CAD build for the part. Positions are in the model's coordinates, mm. Face numbers are marked on the shaded views. A direction names the side the tool comes from. Round coordinates to 2 decimals unless told otherwise and drop trailing zeros. Loops run counter-clockwise (first coordinate to the right, second up) from the corner with the lowest first, then second, coordinate; pieces in that order, holes last. Notation, with made-up numbers: M 23.25,83.5 L 62.25,83.5 A17 cw 62.25,109.5 Z; hole C -27.75,68.25 d2. An arc over 180 degrees is marked long. Use one line per item in the form item = value.
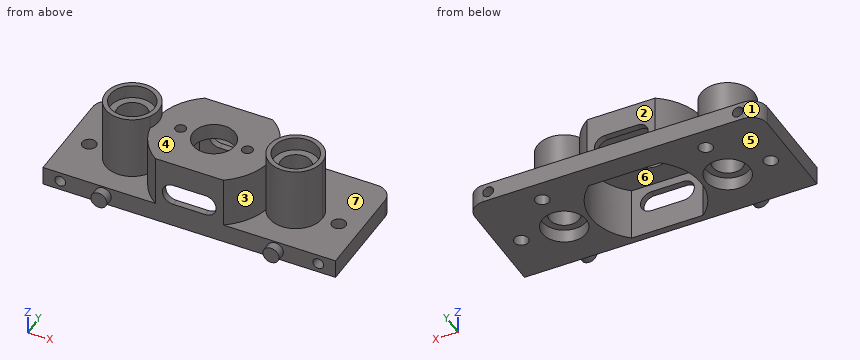
from build123d import *

# Parameters (mm, degrees)
SKETCH_2_R               = 3.9
SKETCH_2_R_2             = 4.1
SKETCH_2_R_3             = 1
SKETCH_2_R_4             = 1.3
EXTRUDE_1_DEPTH          = 3.5
SKETCH_2_4_R             = 4.1
SKETCH_2_4_R_2           = 2.8
EXTRUDE_2_DEPTH          = 1
CUT_EXTRUDE_1_DEPTH      = 41.636067723
CUT_EXTRUDE_1_DEPTH_BACK = 41.636067723
SKETCH_3_W               = 54.4
SKETCH_3_H               = 21
FILLET_1_R               = 3
CUT_EXTRUDE_2_DEPTH      = 35.541134897
CUT_EXTRUDE_2_DEPTH_BACK = 7
SKETCH_4_R               = 1
SKETCH_4_4_R             = 1.5
EXTRUDE_3_DEPTH          = 1.6
SKETCH_5_R               = 1
SKETCH_5_R_2             = 3.9
EXTRUDE_4_DEPTH          = 13
SKETCH_6_R               = 1
SKETCH_6_R_2             = 3.9
CUT_EXTRUDE_3_DEPTH      = 10
CUT_EXTRUDE_4_DEPTH      = 36.958309193
CUT_EXTRUDE_4_DEPTH_BACK = 36.958309193
SKETCH_2_5_R             = 4.1
SKETCH_2_5_R_2           = 2.8
EXTRUDE_5_DEPTH          = 13
SKETCH_8_R               = 4.1
EXTRUDE_6_DEPTH          = 12
EXTRUDE_START            = 9.5
EXTRUDE_7_DEPTH          = 2.5
SKETCH_2_6_R             = 4.1
SKETCH_2_6_R_2           = 2.8
CUT_EXTRUDE_10_DEPTH     = 2.5
SKETCH_9_R               = 1
CUT_EXTRUDE_11_DEPTH     = 6


# Read off the part's stored shape, not the designer's step: 凸台-拉伸7
with BuildPart() as part:
    # 草图2 → 凸台-拉伸1 (new body)
    with BuildSketch(Plane.XY):
        with BuildLine():
            Line((15.2, -20), (-15.2, -20))
            ThreePointArc((-15.2, -20), (-35.2, 0), (-15.2, 20))
            Line((-15.2, 20), (15.2, 20))
            ThreePointArc((15.2, 20), (35.2, 0), (15.2, -20))
        make_face()
        Circle(SKETCH_2_R, mode=Mode.SUBTRACT)
        with Locations((-15.2, 0)):
            Circle(SKETCH_2_R_2, mode=Mode.SUBTRACT)
        with Locations((15.2, 0)):
            Circle(SKETCH_2_R_2, mode=Mode.SUBTRACT)
        with Locations((-6.2, 0)):
            Circle(SKETCH_2_R_3, mode=Mode.SUBTRACT)
        with Locations((6.2, 0)):
            Circle(SKETCH_2_R_3, mode=Mode.SUBTRACT)
        with Locations((-15.2, 8)):
            Circle(SKETCH_2_R_4, mode=Mode.SUBTRACT)
        with Locations((-23.2, 0)):
            Circle(SKETCH_2_R_4, mode=Mode.SUBTRACT)
        with Locations((23.2, 0)):
            Circle(SKETCH_2_R_4, mode=Mode.SUBTRACT)
        with Locations((15.2, 8)):
            Circle(SKETCH_2_R_4, mode=Mode.SUBTRACT)
    extrude(amount=EXTRUDE_1_DEPTH)

    # 草图2<4> → 凸台-拉伸2 (add)
    # profile 1 of 2: a face of its own
    with BuildSketch(Plane.XY):
        with Locations((-15.2, 0)):
            Circle(SKETCH_2_4_R)
        with Locations((-15.2, 0)):
            Circle(SKETCH_2_4_R_2, mode=Mode.SUBTRACT)
    # profile 2 of 2: a face of its own
    with BuildSketch(Plane.XY):
        with Locations((15.2, 0)):
            Circle(SKETCH_2_4_R)
        with Locations((15.2, 0)):
            Circle(SKETCH_2_4_R_2, mode=Mode.SUBTRACT)
    extrude(amount=EXTRUDE_2_DEPTH)

    # 草图3 → 切除-拉伸1 (cut, two sides: drawn at the far end of the back side and taken through both)
    with BuildSketch(Plane.XY.offset(3.5).offset(-CUT_EXTRUDE_1_DEPTH_BACK)):
        with BuildLine():
            Line((15.2, -20), (-15.2, -20))
            ThreePointArc((-15.2, -20), (-35.2, 0), (-15.2, 20))
            Line((-15.2, 20), (15.2, 20))
            ThreePointArc((15.2, 20), (35.2, 0), (15.2, -20))
        make_face()
        with Locations((0, 1.5)):
            Rectangle(SKETCH_3_W, SKETCH_3_H, mode=Mode.SUBTRACT)
    extrude(amount=CUT_EXTRUDE_1_DEPTH + CUT_EXTRUDE_1_DEPTH_BACK, mode=Mode.SUBTRACT)

    # 圆角1
    fillet_1_edges = [part.edges().sort_by_distance(p)[0] for p in [
        (27.2, 12, 1.75),
        (-27.2, 12, 1.75),
    ]]
    fillet(fillet_1_edges, radius=FILLET_1_R)

    # 草图4 → 切除-拉伸2 (cut, two sides: drawn at the far end of the back side and taken through both)
    with BuildSketch(Plane.XZ.offset(9).offset(-CUT_EXTRUDE_2_DEPTH_BACK)):
        with Locations(Location((-24, 1.75, 0), (0, 0, 90))):
            Circle(SKETCH_4_R)
        with Locations(Location((24, 1.75, 0), (0, 0, 90))):
            Circle(SKETCH_4_R)
    extrude(amount=CUT_EXTRUDE_2_DEPTH + CUT_EXTRUDE_2_DEPTH_BACK, mode=Mode.SUBTRACT)

    # 草图4<4> → 凸台-拉伸3 (add)
    with BuildSketch(Plane.XZ.offset(9)):
        with Locations(Location((-16, 1.75, 0), (0, 0, 270))):
            Circle(SKETCH_4_4_R)
        with Locations(Location((16, 1.75, 0), (0, 0, 270))):
            Circle(SKETCH_4_4_R)
    extrude(amount=EXTRUDE_3_DEPTH)

    # 草图5 → 凸台-拉伸4 (add)
    with BuildSketch(Plane(origin=(0, 0, 0), x_dir=(-1, 0, 0), z_dir=(0, 0, -1))):
        with BuildLine():
            Line((6.32455532, 9), (-6.32455532, 9))
            ThreePointArc((-6.32455532, 9), (-11, 0), (-6.32455532, -9))
            Line((-6.32455532, -9), (6.32455532, -9))
            ThreePointArc((6.32455532, -9), (9.761406367, -5.070990607), (11, 0))
            ThreePointArc((11, 0), (9.761406367, 5.070990607), (6.32455532, 9))
        make_face()
        with Locations((-6.2, 0)):
            Circle(SKETCH_5_R, mode=Mode.SUBTRACT)
        Circle(SKETCH_5_R_2, mode=Mode.SUBTRACT)
        with Locations((6.2, 0)):
            Circle(SKETCH_5_R, mode=Mode.SUBTRACT)
    extrude(amount=-EXTRUDE_4_DEPTH)

    # 草图6 → 切除-拉伸3 (cut)
    with BuildSketch(Plane(origin=(0, 0, 0), x_dir=(-1, 0, 0), z_dir=(0, 0, -1))):
        with BuildLine():
            Line((6.65, 7.8), (-6.65, 7.8))
            ThreePointArc((-6.65, 7.8), (-10.25, 0), (-6.65, -7.8))
            Line((-6.65, -7.8), (6.65, -7.8))
            ThreePointArc((6.65, -7.8), (9.306583691, -4.295346319), (10.25, 0))
            ThreePointArc((10.25, 0), (9.306583691, 4.295346319), (6.65, 7.8))
        make_face()
        with Locations((-6.2, 0)):
            Circle(SKETCH_6_R, mode=Mode.SUBTRACT)
        Circle(SKETCH_6_R_2, mode=Mode.SUBTRACT)
        with Locations((6.2, 0)):
            Circle(SKETCH_6_R, mode=Mode.SUBTRACT)
    extrude(amount=-CUT_EXTRUDE_3_DEPTH, mode=Mode.SUBTRACT)

    # 草图7 → 切除-拉伸4 (cut, two sides: drawn at the far end of the back side and taken through both)
    with BuildSketch(Plane(origin=(0, 9, 0), x_dir=(1, 0, 0), z_dir=(0, 1, 0)).offset(-CUT_EXTRUDE_4_DEPTH_BACK)):
        with BuildLine():
            Line((-3, -4.5), (3, -4.5))
            ThreePointArc((3, -4.5), (5, -6.5), (3, -8.5))
            Line((3, -8.5), (-3, -8.5))
            ThreePointArc((-3, -8.5), (-5, -6.5), (-3, -4.5))
        make_face()
    extrude(amount=CUT_EXTRUDE_4_DEPTH + CUT_EXTRUDE_4_DEPTH_BACK, mode=Mode.SUBTRACT)

    # 草图2<5> → 凸台-拉伸5 (add)
    # profile 1 of 2: a face of its own
    with BuildSketch(Plane.XY):
        with Locations(Location((-15.2, 0, 0), (0, 0, 180))):
            Circle(SKETCH_2_5_R)
        with Locations((-15.2, 0)):
            Circle(SKETCH_2_5_R_2, mode=Mode.SUBTRACT)
    # profile 2 of 2: a face of its own
    with BuildSketch(Plane.XY):
        with Locations(Location((15.2, 0, 0), (0, 0, 180))):
            Circle(SKETCH_2_5_R)
        with Locations((15.2, 0)):
            Circle(SKETCH_2_5_R_2, mode=Mode.SUBTRACT)
    extrude(amount=EXTRUDE_5_DEPTH)

    # 草图8 → 凸台-拉伸6 (add)
    # profile 1 of 2: a face of its own
    with BuildSketch(Plane.XY.offset(3.5)):
        with BuildLine():
            ThreePointArc((-10.774259868, -2.217053064), (-11, 0), (-10.774259868, 2.217053064))
            ThreePointArc((-10.774259868, 2.217053064), (-20.15, 0), (-10.774259868, -2.217053064))
        make_face()
        with Locations((-15.2, 0)):
            Circle(SKETCH_8_R, mode=Mode.SUBTRACT)
    # profile 2 of 2: a face of its own
    with BuildSketch(Plane.XY.offset(3.5)):
        with BuildLine():
            ThreePointArc((10.774259868, -2.217053064), (16.339097526, -4.817152356), (20.15, 0))
            ThreePointArc((20.15, 0), (16.339097526, 4.817152356), (10.774259868, 2.217053064))
            ThreePointArc((10.774259868, 2.217053064), (11, 0), (10.774259868, -2.217053064))
        make_face()
        with Locations((15.2, 0)):
            Circle(SKETCH_8_R, mode=Mode.SUBTRACT)
    extrude(amount=EXTRUDE_6_DEPTH)

    # 凸台-拉伸7 outline → 凸台-拉伸7 (add)
    with BuildSketch(Plane.XY.offset(3.5).offset(EXTRUDE_START)):
        with BuildLine():
            ThreePointArc((-10.774259868, -2.217053064), (-10.25, 0), (-10.774259868, 2.217053064))
            ThreePointArc((-10.774259868, 2.217053064), (-11, 0), (-10.774259868, -2.217053064))
        make_face()
        with BuildLine():
            ThreePointArc((10.774259868, -2.217053064), (11, 0), (10.774259868, 2.217053064))
            ThreePointArc((10.774259868, 2.217053064), (10.25, 0), (10.774259868, -2.217053064))
        make_face()
    extrude(amount=EXTRUDE_7_DEPTH)

    # 草图2<6> → 切除-拉伸10 (cut)
    # profile 1 of 2: a face of its own
    with BuildSketch(Plane.XY):
        with Locations((-15.2, 0)):
            Circle(SKETCH_2_6_R)
        with Locations((-15.2, 0)):
            Circle(SKETCH_2_6_R_2, mode=Mode.SUBTRACT)
    # profile 2 of 2: a face of its own
    with BuildSketch(Plane.XY):
        with Locations((15.2, 0)):
            Circle(SKETCH_2_6_R)
        with Locations((15.2, 0)):
            Circle(SKETCH_2_6_R_2, mode=Mode.SUBTRACT)
    extrude(amount=CUT_EXTRUDE_10_DEPTH, mode=Mode.SUBTRACT)

    # 草图9 → 切除-拉伸11 (cut)
    with BuildSketch(Plane(origin=(0, 12, 0), x_dir=(1, 0, 0), z_dir=(0, 1, 0))):
        with Locations(Location((-23.2, -1.75, 0), (0, 0, 270))):
            Circle(SKETCH_9_R)
        with Locations(Location((23.2, -1.75, 0), (0, 0, 270))):
            Circle(SKETCH_9_R)
    extrude(amount=-CUT_EXTRUDE_11_DEPTH, mode=Mode.SUBTRACT)


solid = part.part
1. Cut at D-D on y = 10.75. Write the cut outline in (x, z).
Completed:
outline = M -26.64,0 L 26.64,0 L 26.64,3.5 L -26.64,3.5 Z; hole C -23.2,1.75 d2; hole C 23.2,1.75 d2
2. Cut at A-A on x = 0. Write the cut outline in (y, z).
Completed:
outline = M -9,0 L -7.8,0 L -7.8,4.5 L -9,4.5 Z; M -9,8.5 L -7.8,8.5 L -7.8,10 L -3.9,10 L -3.9,13 L -9,13 Z; M 3.9,10 L 7.8,10 L 7.8,8.5 L 9,8.5 L 9,13 L 3.9,13 Z; M 7.8,0 L 12,0 L 12,3.5 L 9,3.5 L 9,4.5 L 7.8,4.5 Z
3. Cut at C-C on z = 10.75. Write the cut outline in (x, y).
Completed:
outline = M -10.77,-2.22 A11 ccw -6.32,-9 L 6.32,-9 A11 ccw 10.77,-2.22 A4.95 ccw long 10.77,2.22 A11 ccw 6.32,9 L -6.32,9 A11 ccw -10.77,2.22 A4.95 ccw long Z; hole C -15.2,0 d5.6; hole C -6.2,0 d2; hole C 0,0 d7.8; hole C 6.2,0 d2; hole C 15.2,0 d5.6
4. Drop flat-ended pins along their axis: P1, Ø2, axis at x = 17.5, z = 11.5, coming from the -Y side; P2, Ø7.5, axis at x = -15.2, y = 0, coming from the +Z side; P3, Ø4, axis at x = -15.2, y = 8, coming from the +Z side. Give the stop position or say it passes through.
Completed:
P1 = -4.78
P2 = 13
P3 = 3.5
5. Tool access for the marked faces 5, 6 and 7: list every direction of +Z, -Z, +X, -X, +Y, -Y with a clear straight run to the whole face (end or side of a thin tool).
Completed:
face_5 = -Z, +X, -X, +Y, -Y
face_6 = -Z
face_7 = +Z
6. Cut at B-B on z = 5. Write the cut outline in (x, y), and give its area (3 significant figures).
Completed:
outline = M -10.77,-2.22 A11 ccw -6.32,-9 L -4.32,-9 L -4.32,-7.8 L -6.65,-7.8 A10.25 cw -6.65,7.8 L -4.32,7.8 L -4.32,9 L -6.32,9 A11 ccw -10.77,2.22 A4.95 ccw long Z; M 4.32,-9 L 6.32,-9 A11 ccw 10.77,-2.22 A4.95 ccw long 10.77,2.22 A11 ccw 6.32,9 L 4.32,9 L 4.32,7.8 L 6.65,7.8 A10.25 cw 6.65,-7.8 L 4.32,-7.8 Z; hole C -15.2,0 d5.6; hole C 15.2,0 d5.6
area = 140 mm2
7. Probe line 1 along Y through (x, z) = (-6, 5.5); line 2 along X through (y, z) = (4.5, 5); line 3 along Z through (x, y) = (24, -6). List the from-to ranges inside material, lowest first. Write a range as from..to.
Completed:
line_1 = -9..-7.8, 7.8..9
line_2 = -17.26..-13.14, -10.04..-9.21, 9.21..10.04, 13.14..17.26
line_3 = 0..0.75, 2.75..3.5
8. Pull direction X, two halves, no side cores. Call the marked faces 1, 2, 3 and 4: +X half, -X half, draft (parallel to the pull), parting line (faces both ways), or undercut.
Completed:
face_1 = -X half
face_2 = draft
face_3 = undercut
face_4 = undercut
